Geometry: final body of the model. Coordinates: model frame, mm. Give positions to 0.01 mm unless a question says otherwise; leave off trailing zeros. Loops run counter-clockwise (first coordinate to the right, second up) from the corner with the lowest first, then second, coordinate; pieces in that order, holes last. Notation, with made-up numbers: M -37,-13 L 5,-13 A23 ccw 5,13 Z; hole C -31.75,64.25 d6. An arc over 180 degrees is marked long. Put each result on its own line as item: value.
```python
from build123d import *

# Parameters (mm, degrees)
SALIENTE_EXTRUIR1_DEPTH      = 3
TALADRO_DE_MARGEN_PARA_M51_D = 5.5
CROQUIS7_W                   = 15
CROQUIS7_H                   = 6
CROQUIS7_W_2                 = 6
CROQUIS7_H_2                 = 15
CORTAR_EXTRUIR1_DEPTH        = 145.086779407


with BuildPart() as part:
    # Croquis1 → Saliente-Extruir1 (new, symmetric)
    with BuildSketch(Plane(origin=(0, 0, 0), x_dir=(1, 0, 0), z_dir=(0, 1, 0))):
        with BuildLine():
            Line((-40, 50), (85, 50))
            ThreePointArc((85, 50), (135, 0), (85, -50))
            Line((85, -50), (-40, -50))
            ThreePointArc((-40, -50), (-90, 0), (-40, 50))
        make_face()
    extrude(amount=SALIENTE_EXTRUIR1_DEPTH, both=True)

    # Taladro de margen para M51 (through all)
    with Locations(Plane(origin=(0, 3, 0), x_dir=(1, 0, 0), z_dir=(0, 1, 0))):
        with Locations((0, 0)):
            Hole(TALADRO_DE_MARGEN_PARA_M51_D / 2)

    # Croquis7 → Cortar-Extruir1 (cut, through all)
    with BuildSketch(Plane(origin=(0, -3, 0), x_dir=(-1, 0, 0), z_dir=(0, -1, 0))):
        with Locations((-87.09375, -25)):
            Rectangle(CROQUIS7_W, CROQUIS7_H)
        with Locations((-112.09375, -25)):
            Rectangle(CROQUIS7_W, CROQUIS7_H)
        with Locations((-112.09375, 25)):
            Rectangle(CROQUIS7_W, CROQUIS7_H)
        with Locations((-87.09375, 25)):
            Rectangle(CROQUIS7_W, CROQUIS7_H)
        with Locations((-76.59375, -12.5)):
            Rectangle(CROQUIS7_W_2, CROQUIS7_H_2)
        with Locations((-76.59375, 12.5)):
            Rectangle(CROQUIS7_W_2, CROQUIS7_H_2)
    cortar_extruir1 = extrude(amount=-CORTAR_EXTRUIR1_DEPTH, mode=Mode.SUBTRACT)

    # Simetría1: Cortar-Extruir1 across plane
    add(cortar_extruir1.mirror(Plane(origin=(21, 0, 0), x_dir=(0, 0, 1), z_dir=(1, 0, 0))), mode=Mode.SUBTRACT)


solid = part.part
```
Item 1: Section D-D on y = 0.3. Count the separate pieces of the cut face and the enclosed holes in it, then the cut area to 3 significant figures.
Output values:
separate pieces: 1
enclosed holes: 13
area: 19,300 mm²
Item 2: Line query: probe 1 along Z at (x, y) = (0, 0.4); probe 2 along X at (y, z) = (-1.15, -26); probe 3 along X at (y, z) = (-2.4, 23). Output: solid intervals per line, ascending. Write a range as [from, to].
Output values:
probe 1: [-50, -2.75], [2.75, 50]
probe 2: [-82.71, -77.59], [-62.59, -52.59], [-37.59, 79.59], [94.59, 104.59], [119.59, 127.71]
probe 3: [-84.4, -77.59], [-62.59, -52.59], [-37.59, 79.59], [94.59, 104.59], [119.59, 129.4]
Item 3: Section C-C on x = -67.5. Output: boundary loops of the cut face in (y, z), then the cut area to 3 significant figures.
Output values:
outline: M -3,-41.76 L 3,-41.76 L 3,-28 L -3,-28 Z; M -3,-22 L 3,-22 L 3,22 L -3,22 Z; M -3,28 L 3,28 L 3,41.76 L -3,41.76 Z
area: 429 mm²
Item 4: Mould query, pull axis Z, two halves, no side actions, for faces 1 (the cylindrical face through (-89.988, 0.042, 1.099)), 2 (the flat face through (-52.594, 0, -25)), 3 (the flat face through (22, 0, -50)). Classes: pulls with the +Z half, pulls with the -Z half, needs draft (parallel to the pull), parting line crosses it, or undercut.
Output values:
face 1: parting line crosses it
face 2: undercut
face 3: pulls with the -Z half
Item 5: Pin query (flat end, axial travel): pin 1 Ø1.8 at (y, z) = (-1, -14.5) entering from +X; pin 2 Ø3 at (y, z) = (1.5, -25) entering from -X; pin 3 Ø2 at (y, z) = (1.5, -40) entering from +X. Return the tip coordinate at first contact, or that it passes through.
Output values:
pin 1: x = 133.11
pin 2: x = -84.13
pin 3: x = 116.29
Item 6: Section B-B on z = -7.5. Output: boundary loops of the cut face in (x, y).
Output values:
outline: M -89.43,-3 L -37.59,-3 L -37.59,3 L -89.43,3 Z; M -31.59,-3 L 73.59,-3 L 73.59,3 L -31.59,3 Z; M 79.59,-3 L 134.43,-3 L 134.43,3 L 79.59,3 Z
Item 7: Section A-A on x = 0. Output: boundary loops of the cut face in (y, z), then the cut area to 3 significant figures.
Output values:
outline: M -3,-50 L 3,-50 L 3,-2.75 L -3,-2.75 Z; M -3,2.75 L 3,2.75 L 3,50 L -3,50 Z
area: 567 mm²
